Here's the drawing with two shaded views (mm, measured from the low corner). I have some questions. A direction names the side the tool comes from. Give positions to 0.01 mm unless a question says otherwise; leave off trailing zeros. Loops run counter-clockwise (first coordinate to the right, second up) from the corner with the lowest first, then second, coordinate; pieces in that order, holes last. Notation, with made-up numbers: M 24,22 L 42,22 A18 ccw 42,44 Z; hole C 35.25,67 d7. An arc over 180 degrees is marked long. Write item = value, one per line. Start each with the question number.
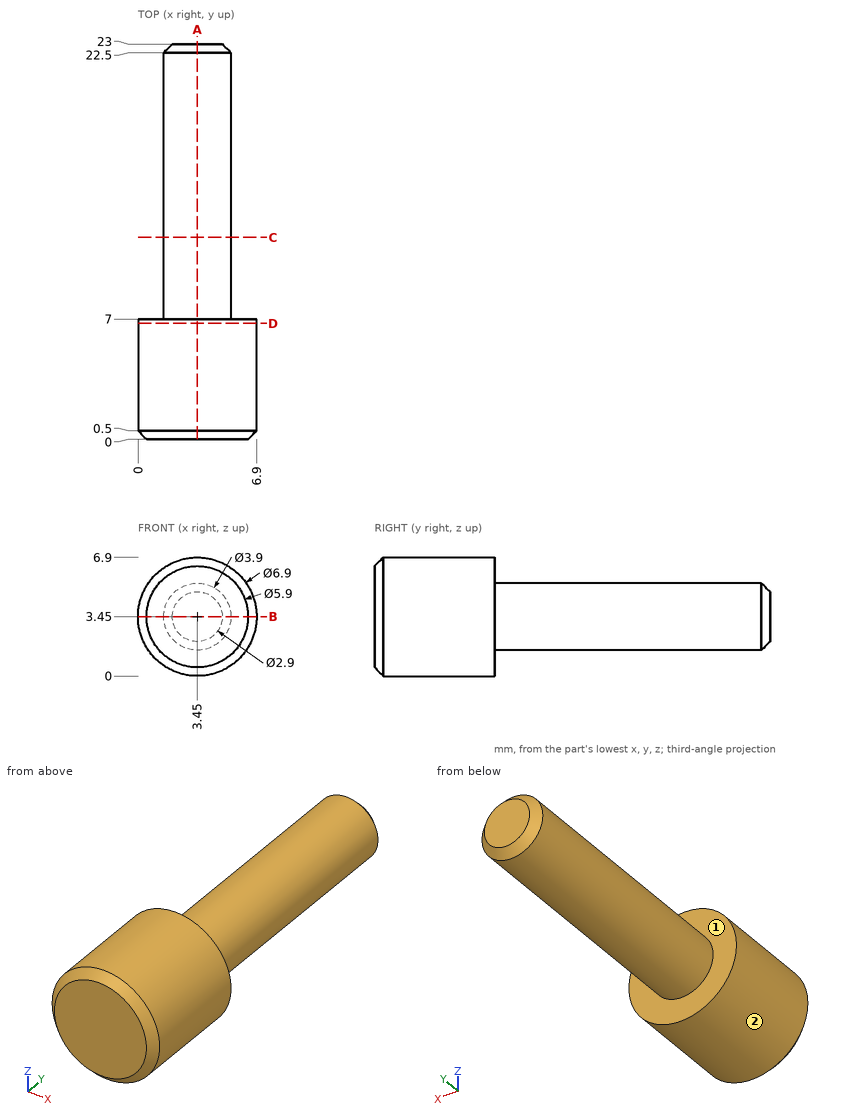
Q1. On a 3-axis mill with a long thin cutter (end or side, diameter ignored), from which of +Z, -Z, +X, -X, +Y, -Y can I reach the whole of each face in a straight line? I mean the marked faces 1 and 2. Say none if no direction works.
Q2. Will these pins go through, and if not, where does the flat tip stop? pin 1 (2 mm diameter, centred on x = 1, y = 18.5, fed in from -Z); pin 2 (2 mm diameter, centred on x = 4, y = 8.5, fed in from +Z); pin 3 (2 mm diameter, centred on y = 12.5, z = 3.5, fed in from +X).
Q3. If I drill on line 1 along Y through (x, z) = (1.75, 5.75); line 2 along Z through (x, y) = (3.5, 9.75); line 3 along X through (y, z) = (7.25, 4), over which ranges is the centre line in solid material (lowest first)?
Q4. If we section it at A-A, the plane x = 3.45: List the corners of the cut face in (y, z) for me, then the cut area to 3 significant figures.
Q5. If we section it at D-D, the plane y = 6.75: List the corners of the cut face in (x, z) for me.
Q6. If we section it at B-B, the plane z = 3.45: List the corners of the cut face in (x, y) for me, then the cut area to 3 significant figures.
Q7. If we section it at C-C, the plane y = 11.75: List the corners of the cut face in (x, z) for me.
Resolved:
q1.face_1 = +Y
q1.face_2 = +Y, -Y
q2.pin_1 = 2.15
q2.pin_2 = 5.4
q2.pin_3 = 5.4
q3.line_1 = 0 to 7
q3.line_2 = 1.5 to 5.4
q3.line_3 = 1.58 to 5.32
q4.outline = M 0,0.5 L 0.5,0 L 7,0 L 7,1.5 L 22.5,1.5 L 23,2 L 23,4.9 L 22.5,5.4 L 7,5.4 L 7,6.9 L 0.5,6.9 L 0,6.4 Z
q4.area = 110 mm²
q5.outline = C 3.45,3.45 d6.9
q6.outline = M 0,0.5 L 0.5,0 L 6.4,0 L 6.9,0.5 L 6.9,7 L 5.4,7 L 5.4,22.5 L 4.9,23 L 2,23 L 1.5,22.5 L 1.5,7 L 0,7 Z
q6.area = 110 mm²
q7.outline = C 3.45,3.45 d3.9
